The listing builds one solid part. Answer for the finished solid, in the listing's coordinates (mm). Face numbers are marked on the shaded views. A direction names the side the tool comes from. Give positions to 0.01 mm unless a question says otherwise; leave off trailing zeros. Order: outer loops, then holes, each group sorted by start corner. A loop starts at its lowest first (then second) coordinate and runs counter-clockwise, first axis right, second up. Notation, with made-up numbers: (89, -36) - (117, -36) arc R21 cw to (117, -27) - close; hole circle Ø1 at (1.25, 43). An arc over 180 degrees is marked (long way). Use a Markdown table: item, result. Add a question column.
1) Find section D-D, the plane z = 14.5. Determine the outline of the cut face in (x, y).
2) For the marked faces 1, 2 and 3, determine the directions among +Z, -Z, +X, -X, +Y, -Y from which every point of the face is accessible in a straight line to the end or side of a thin tool.
3) Find section B-B, the plane y = 0. Determine the outline of the cut face in (x, z), plus the area to 3 significant figures.
4) Flat-ended cylindrical pins translate along their axes: pin 1 (4 mm diameter, centred on x = 6, y = 5, fed in from +Z); pin 2 (6 mm diameter, centred on y = 3, z = 18, fed in from -X); pin 3 (8 mm diameter, centred on x = -5.5, z = 8, fed in from +Y). Find the tip coordinate at first contact, or state that the pin passes through.
5) Find section A-A, the plane x = 0. Determine the outline of the cut face in (y, z).
6) Straight lines are drawn through the part: line 1 (Z direction, x = -1, y = 0); line 2 (Z direction, x = 6.75, y = -0.25); line 3 (Y direction, x = 1.75, z = 22.5). For each, find the intervals that lie inside material, in ascending order.
7) Find section C-C, the plane z = 22.5. Determine the outline of the cut face in (x, y), plus the area to 3 significant figures.
from build123d import *

# Parameters (mm, degrees)
F0_R     = 4
F1_DEPTH = 26
F3_R     = 7.5
F4_DEPTH = 5
F5_R     = 1.25
F6_DEPTH = 12.5


with BuildPart() as f1:
    # F0 (on Top) → F1 (new body)
    with BuildSketch(Plane.XY):
        Circle(F0_R)
    extrude(amount=F1_DEPTH)

    # F3 (on offset) → F4 (join)
    with BuildSketch(Plane(origin=(0, 0, 8), x_dir=(1, 0, 0), z_dir=(0, 0, -1))):
        Circle(F3_R)
    extrude(amount=-F4_DEPTH)

    # F5 (on Right) → F6 (cut, symmetric)
    with BuildSketch(Plane.YZ):
        with Locations((0, 22.5)):
            Circle(F5_R)
    extrude(amount=F6_DEPTH, both=True, mode=Mode.SUBTRACT)


solid = f1.part
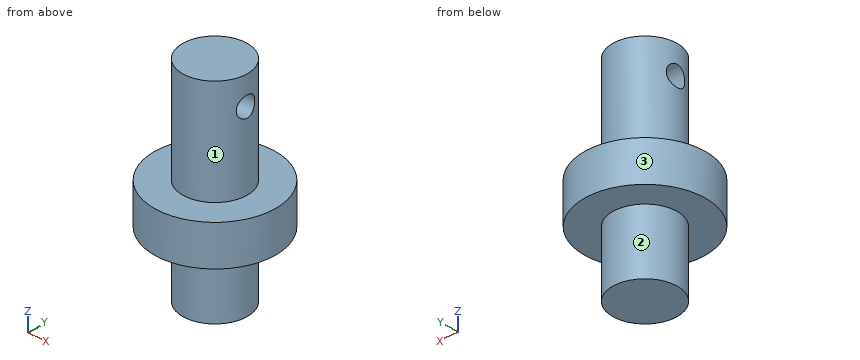
The answers:
| question | item | result |
|---|---|---|
| 1 | outline | circle Ø8 at (0, 0) |
| 2 | face 1 | +Z |
| 2 | face 2 | -Z |
| 2 | face 3 | +Z, -Z |
| 3 | outline | (-7.5, 8) - (-4, 8) - (-4, 0) - (4, 0) - (4, 8) - (7.5, 8) - (7.5, 13) - (4, 13) - (4, 21.25) - (-4, 21.25) - (-4, 13) - (-7.5, 13) - close; (-4, 23.75) - (4, 23.75) - (4, 26) - (-4, 26) - close |
| 3 | area | 223 mm2 |
| 4 | pin 1 | z = 13 |
| 4 | pin 2 | x = -4 |
| 4 | pin 3 | y = 7.35 |
| 5 | outline | (-7.5, 8) - (-4, 8) - (-4, 0) - (4, 0) - (4, 8) - (7.5, 8) - (7.5, 13) - (4, 13) - (4, 26) - (-4, 26) - (-4, 13) - (-7.5, 13) - close; hole circle Ø2.5 at (0, 22.5) |
| 6 | line 1 | 0 to 21.25, 23.75 to 26 |
| 6 | line 2 | 8 to 13 |
| 6 | line 3 | -3.6 to -1.25, 1.25 to 3.6 |
| 7 | outline | (-3.8, -1.25) arc R4 ccw to (3.8, -1.25) - close; (-3.8, 1.25) - (3.8, 1.25) arc R4 ccw to start |
| 7 | area | 30.6 mm2 |
